from build123d import *

# Parameters (mm, degrees)
SKETCH1_W           = 66
SKETCH1_H           = 25
BOSS_EXTRUDE1_DEPTH = 4
SKETCH2_W           = 4
SKETCH2_H           = 5
BOSS_EXTRUDE2_DEPTH = 4
LPATTERN1_COUNT     = 2
LPATTERN1_PITCH     = 10
SKETCH3_W           = 10
SKETCH3_H           = 4
BOSS_EXTRUDE3_DEPTH = 4
LPATTERN2_COUNT     = 2
LPATTERN2_PITCH     = 20
LPATTERN2_COL_COUNT = 2
LPATTERN2_COL_PITCH = 20
SKETCH4_W           = 10
SKETCH4_H           = 4
CUT_EXTRUDE1_DEPTH  = 75.437893576
SKETCH8_R           = 1.5
CUT_EXTRUDE4_DEPTH  = 75.437893576


with BuildPart() as part:
    # Sketch1 → Boss-Extrude1 (new body)
    with BuildSketch(Plane(origin=(0, 0, 0), x_dir=(1, 0, 0), z_dir=(0, 1, 0))):
        with Locations((33, -12.5)):
            Rectangle(SKETCH1_W, SKETCH1_H)
    extrude(amount=BOSS_EXTRUDE1_DEPTH)

    # Sketch2 → Boss-Extrude2 (add, through all)
    with BuildSketch(Plane(origin=(0, 4, 0), x_dir=(1, 0, 0), z_dir=(0, 1, 0))):
        with Locations((-2, -17.5)):
            Rectangle(SKETCH2_W, SKETCH2_H)
        with Locations((68, -17.5)):
            Rectangle(SKETCH2_W, SKETCH2_H)
    boss_extrude2 = extrude(amount=-BOSS_EXTRUDE2_DEPTH)

    # LPattern1: Boss-Extrude2 ×2
    with Locations(*[(0, 0, -i * LPATTERN1_PITCH) for i in range(1, LPATTERN1_COUNT)]):
        add(boss_extrude2)

    # Sketch3 → Boss-Extrude3 (add, through all)
    with BuildSketch(Plane(origin=(0, 4, 0), x_dir=(1, 0, 0), z_dir=(0, 1, 0))):
        with Locations((33, 2)):
            Rectangle(SKETCH3_W, SKETCH3_H)
    boss_extrude3 = extrude(amount=-BOSS_EXTRUDE3_DEPTH)

    # LPattern2: Boss-Extrude3 ×2
    with Locations(*[(i * LPATTERN2_PITCH, 0, 0) for i in range(1, LPATTERN2_COUNT)]):
        add(boss_extrude3)

    # LPattern2 col: Boss-Extrude3 ×2
    with Locations(*[(-i * LPATTERN2_COL_PITCH, 0, 0) for i in range(1, LPATTERN2_COL_COUNT)]):
        add(boss_extrude3)

    # Sketch4 → Cut-Extrude1 (cut, through all)
    with BuildSketch(Plane.XZ):
        with Locations((13, 6)):
            Rectangle(SKETCH4_W, SKETCH4_H)
        with Locations((33, 6)):
            Rectangle(SKETCH4_W, SKETCH4_H)
        with Locations((53, 6)):
            Rectangle(SKETCH4_W, SKETCH4_H)
    extrude(amount=-CUT_EXTRUDE1_DEPTH, mode=Mode.SUBTRACT)

    # Sketch8 → Cut-Extrude4 (cut, through all)
    with BuildSketch(Plane(origin=(0, 4, 0), x_dir=(1, 0, 0), z_dir=(0, 1, 0))):
        with Locations(Location((51.5, -13, 0), (0, 0, 270))):
            Circle(SKETCH8_R)
        with Locations(Location((46.5, -13, 0), (0, 0, 270))):
            Circle(SKETCH8_R)
        with Locations(Location((40, -13, 0), (0, 0, 270))):
            Circle(SKETCH8_R)
        with Locations(Location((35, -13, 0), (0, 0, 270))):
            Circle(SKETCH8_R)
        with Locations(Location((30, -13, 0), (0, 0, 270))):
            Circle(SKETCH8_R)
        with Locations(Location((23.5, -13, 0), (0, 0, 270))):
            Circle(SKETCH8_R)
        with Locations(Location((18.5, -13, 0), (0, 0, 270))):
            Circle(SKETCH8_R)
        with Locations(Location((13.5, -13, 0), (0, 0, 270))):
            Circle(SKETCH8_R)
    extrude(amount=-CUT_EXTRUDE4_DEPTH, mode=Mode.SUBTRACT)


solid = part.part
Could you check a few things on this model? Use its own coordinates, in mm. A direction names the side the tool comes from. Give positions to 0.01 mm unless a question says otherwise; leave off trailing zeros. Write each loop counter-clockwise with the first axis right and the second up, starting at its lowest first coordinate (ties: lowest second). Pieces come first, ordered by that corner, then holes. Notation, with made-up numbers: (-2, 31) -> (39, 31) arc R10 cw to (39, 43) -> close; hole circle Ø9 at (70, 6). An arc over 180 degrees is marked (long way). Answer as a JSON object with one key per item and string values.
Q1. Suppose I cut it at A-A on x = 23.5. Write out the boundary of the cut face in (y, z), then the cut area to 3 significant figures.
Taken from the geometry:
{"outline": "(0, 0) -> (4, 0) -> (4, 11.5) -> (0, 11.5) -> close; (0, 14.5) -> (4, 14.5) -> (4, 25) -> (0, 25) -> close", "area": "88.0 mm²"}
Q2. Suppose I cut it at C-C on z = 13. Count the separate pieces of the cut face and the enclosed holes in it, then the cut area to 3 significant figures.
Taken from the geometry:
{"separate pieces": "9", "enclosed holes": "0", "area": "168 mm²"}
Q3. We'd pull the mould along Z, two halves only. Please class faces 6 (the flat face through (66, 2, 23)), 7 (the cylindrical face through (45, 2, 13)), 8 (the flat face through (4, 2, 0)): released by +Z, released by -Z, zero draft, split by the parting line, or undercut.
Taken from the geometry:
{"face 6": "zero draft", "face 7": "undercut", "face 8": "released by -Z"}
Q4. Which directions (+Z, -Z, +X, -X, +Y, -Y) give clear straight access to the entire face, cutting with the end or side of a thin tool? Please do faces 1 (the flat face through (68, 2, 5)), 2 (the flat face through (58, 2, 6)), 3 (the flat face through (0, 2, 13)), 4 (the flat face through (68, 2, 15)), 5 (the flat face through (18, 2, -2)).
Taken from the geometry:
{"face 1": "-Z, +X, +Y, -Y", "face 2": "+Y, -Y", "face 3": "-X, +Y, -Y", "face 4": "+X, +Y, -Y", "face 5": "-Z, +Y, -Y"}
Q5. Will these pins go through, and if not, where does the flat tip stop? pin 1 Ø1.5 at (y, z) = (1.5, 11.5) entering from -X; pin 2 Ø1.2 at (x, y) = (68, 2.5) entering from +Z; pin 3 Ø1.2 at (y, z) = (1.5, -1.5) entering from +X.
Taken from the geometry:
{"pin 1": "stops at x = 0", "pin 2": "stops at z = 20", "pin 3": "stops at x = 58"}
Q6. Suppose I cut it at B-B on x = 51.5. Write out the boundary of the cut face in (y, z), then the cut area to 3 significant figures.
Taken from the geometry:
{"outline": "(0, -4) -> (4, -4) -> (4, 4) -> (0, 4) -> close; (0, 8) -> (4, 8) -> (4, 11.5) -> (0, 11.5) -> close; (0, 14.5) -> (4, 14.5) -> (4, 25) -> (0, 25) -> close", "area": "88.0 mm²"}
Q7. Please list where these lines run through material, in increasing order: L1, parallel to X at y = 0.65, z = 7.5; L2, parallel to Z at x = 14, y = 0.85; L3, parallel to X at y = 0.5, z = 23.25.
Taken from the geometry:
{"L1": "x = -4 to 8, 18 to 28, 38 to 48, 58 to 70", "L2": "z = -4 to 4, 8 to 11.59, 14.41 to 25", "L3": "x = 0 to 66"}
